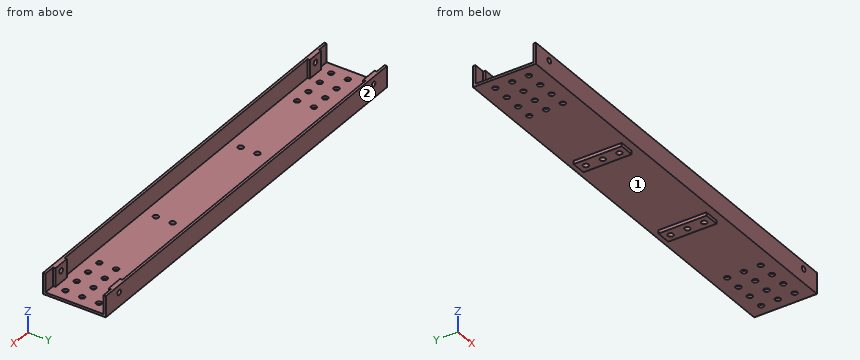
```python
from build123d import *

# Parameters (mm, degrees)
SKETCH_1_W             = 1990
SKETCH_1_H             = 300
SKETCH_1_R             = 13
EXTRUDE_392_DEPTH      = 11.5
EXTRUDE_1_DEPTH        = 89
SKETCH_3_R             = 13
CUT_EXTRUDE_1_DEPTH    = 1045.090633039
PATTERN_LINEAR_1_COUNT = 3
PATTERN_LINEAR_1_PITCH = 80
EXTRUDE_START          = 16
SKETCH_7_W             = 70
SKETCH_7_H             = 230
SKETCH_7_R             = 13
EXTRUDE_2_DEPTH        = 16
SKETCH_8_R             = 12.5
CUT_EXTRUDE_2_DEPTH    = 1045.090633039


with BuildPart() as part:
    # 草图1 → Extrude 392 (new body)
    with BuildSketch(Plane.XY):
        with Locations((0, 150)):
            Rectangle(SKETCH_1_W, SKETCH_1_H)
        with Locations((300, 230)):
            Circle(SKETCH_1_R, mode=Mode.SUBTRACT)
        with Locations((300, 150)):
            Circle(SKETCH_1_R, mode=Mode.SUBTRACT)
        with Locations((300, 70)):
            Circle(SKETCH_1_R, mode=Mode.SUBTRACT)
        with Locations(Location((-300, 70, 0), (0, 0, 180))):
            Circle(SKETCH_1_R, mode=Mode.SUBTRACT)
        with Locations(Location((-300, 150, 0), (0, 0, 180))):
            Circle(SKETCH_1_R, mode=Mode.SUBTRACT)
        with Locations(Location((-300, 230, 0), (0, 0, 180))):
            Circle(SKETCH_1_R, mode=Mode.SUBTRACT)
    extrude(amount=EXTRUDE_392_DEPTH)

    # 草图2 → 凸台-拉伸1 (add)
    with BuildSketch(Plane.XY.offset(11.5)):
        Polygon((-995, 300), (995, 300), (995, 288.5), (940, 288.5), (940, 277.5), (860, 277.5), (860, 288.5), (-860, 288.5), (-860, 277.5), (-940, 277.5), (-940, 288.5), (-995, 288.5), align=None)
        Polygon((-995, 0), (995, 0), (995, 11.5), (940, 11.5), (940, 22.5), (860, 22.5), (860, 11.5), (-860, 11.5), (-860, 22.5), (-940, 22.5), (-940, 11.5), (-995, 11.5), align=None)
    extrude(amount=EXTRUDE_1_DEPTH)

    # 草图3 → 切除-拉伸1 (cut, through all)
    with BuildSketch(Plane(origin=(0, 0, 0), x_dir=(-1, 0, 0), z_dir=(0, 0, -1))):
        with Locations((940, 70)):
            Circle(SKETCH_3_R)
        with Locations((860, 70)):
            Circle(SKETCH_3_R)
        with Locations((780, 70)):
            Circle(SKETCH_3_R)
        with Locations((700, 70)):
            Circle(SKETCH_3_R)
        with Locations((-940, 70)):
            Circle(SKETCH_3_R)
        with Locations((-860, 70)):
            Circle(SKETCH_3_R)
        with Locations((-780, 70)):
            Circle(SKETCH_3_R)
        with Locations((-700, 70)):
            Circle(SKETCH_3_R)
    cut_extrude_1 = extrude(amount=-CUT_EXTRUDE_1_DEPTH, mode=Mode.SUBTRACT)

    # 阵列(线性)1: 切除-拉伸1 ×3
    with Locations(*[(0, i * PATTERN_LINEAR_1_PITCH, 0) for i in range(1, PATTERN_LINEAR_1_COUNT)]):
        add(cut_extrude_1, mode=Mode.SUBTRACT)

    # 草图7 → 凸台-拉伸2 (add)
    # profile 1 of 2: a face of its own
    with BuildSketch(Plane(origin=(0, 0, 0), x_dir=(-1, 0, 0), z_dir=(0, 0, -1)).offset(EXTRUDE_START)):
        with Locations((300, 150)):
            Rectangle(SKETCH_7_W, SKETCH_7_H)
        with Locations((300, 230)):
            Circle(SKETCH_7_R, mode=Mode.SUBTRACT)
        with Locations((300, 150)):
            Circle(SKETCH_7_R, mode=Mode.SUBTRACT)
        with Locations((300, 70)):
            Circle(SKETCH_7_R, mode=Mode.SUBTRACT)
    # profile 2 of 2: a face of its own
    with BuildSketch(Plane(origin=(0, 0, 0), x_dir=(-1, 0, 0), z_dir=(0, 0, -1)).offset(EXTRUDE_START)):
        with Locations((-300, 150)):
            Rectangle(SKETCH_7_W, SKETCH_7_H)
        with Locations(Location((-300, 70, 0), (0, 0, 180))):
            Circle(SKETCH_7_R, mode=Mode.SUBTRACT)
        with Locations(Location((-300, 150, 0), (0, 0, 180))):
            Circle(SKETCH_7_R, mode=Mode.SUBTRACT)
        with Locations(Location((-300, 230, 0), (0, 0, 180))):
            Circle(SKETCH_7_R, mode=Mode.SUBTRACT)
    extrude(amount=-EXTRUDE_2_DEPTH)

    # 草图8 → 切除-拉伸2 (cut, through all)
    with BuildSketch(Plane(origin=(0, 300, 0), x_dir=(-1, 0, 0), z_dir=(0, 1, 0))):
        with Locations(Location((900, 66.5, 0), (0, 0, 90))):
            Circle(SKETCH_8_R)
        with Locations(Location((-900, 66.5, 0), (0, 0, 270))):
            Circle(SKETCH_8_R)
    extrude(amount=-CUT_EXTRUDE_2_DEPTH, mode=Mode.SUBTRACT)


solid = part.part
```
The model under review builds one solid part; all positions refer to its coordinate system, in mm. Face numbers are marked on the shaded views. Give positions to 0.01 mm unless a question says otherwise; leave off trailing zeros. Write each loop counter-clockwise with the first axis right and the second up, starting at its lowest first coordinate (ties: lowest second). Pieces come first, ordered by that corner, then holes.
(1) For P1, Ø1.5, axis at x = 17.5, z = 83.5, coming from the -Y side; P2, Ø9, axis at y = 282.5, z = 40.5, coming from the +X side; P3, Ø12, axis at x = 234.5, y = 155.5, coming from the +Z side, all flat-tipped, find the tip position at first contact; note any pin that passes through.
(2) Consider section A-A, the plane x = 471.5. Give the boundary of the cut face in (y, z), and give its area (3 significant figures).
(3) To check wall thickness, follow L1, parallel to Y at x = -300, z = 5; L2, parallel to X at y = 6, z = 66; L3, parallel to Y at x = -249, z = 51. State the ranges of each line that lie inside material, in increasing order.
(4) The part is to be moulded in two halves that separate along X. For the marked faces 1 and 2, say which applies: released by +X, released by -X, zero draft, split by the parting line, or undercut.
Returned:
1. P1: stops at y = 0
1. P2: stops at x = 940
1. P3: stops at z = 11.5
2. outline: (0, 0) - (300, 0) - (300, 100.5) - (288.5, 100.5) - (288.5, 11.5) - (11.5, 11.5) - (11.5, 100.5) - (0, 100.5) - close
2. area: 5,500 mm2
3. L1: y = 0 to 57, 83 to 137, 163 to 217, 243 to 300
3. L2: x = -995 to -912.49, -887.51 to 887.51, 912.49 to 995
3. L3: y = 0 to 11.5, 288.5 to 300
4. face 1: undercut
4. face 2: zero draft
